from build123d import *

# Parameters (mm, degrees)
F1_DEPTH = 40
F3_DEPTH = 40
F5_DEPTH = 40
F7_DEPTH = 2


with BuildPart() as f1:
    # F0 (on Front) → F1 (new body)
    with BuildSketch(Plane.XZ):
        Polygon((-30, -33.600594), (-15, -7.619832), (-45, -7.619832), align=None)
        Polygon((-18.464102, -9.619832), (-30, -29.600594), (-41.535898, -9.619832), align=None, mode=Mode.SUBTRACT)
        Polygon((0, -33.600594), (-15, -7.619832), (-30, -33.600594), align=None)
        Polygon((-3.464102, -31.600594), (-26.535898, -31.600594), (-15, -11.619832), align=None, mode=Mode.SUBTRACT)
        Polygon((0, -33.600594), (15, -7.619832), (-15, -7.619832), align=None)
        Polygon((-11.535898, -9.619832), (11.535898, -9.619832), (0, -29.600594), align=None, mode=Mode.SUBTRACT)
        Polygon((-15, -7.619832), (15, -7.619832), (0, 18.360931), align=None)
        Polygon((-11.535898, -5.619832), (0, 14.360931), (11.535898, -5.619832), align=None, mode=Mode.SUBTRACT)
    extrude(amount=F1_DEPTH)

    # F2 (on face) → F3 (join)
    with BuildSketch(Plane.XZ.offset(40)):
        Polygon((-30, -33.600594), (-45, -7.619832), (-75, -7.619832), (-105, -7.619832), (-90, -33.600594), align=None)
        Polygon((-33.464102, -31.600594), (-88.845299, -31.600594), (-101.535898, -9.619832), (-75, -9.619832), (-46.154701, -9.619832), align=None, mode=Mode.SUBTRACT)
    extrude(amount=-F3_DEPTH)

    # F4 (on face) → F5 (join)
    with BuildSketch(Plane.XZ.offset(40)):
        Polygon((-75, -7.619832), (-90, 18.360931), (-105, -7.619832), align=None)
        Polygon((-101.535898, -5.619832), (-90, 14.360931), (-78.464102, -5.619832), (-90, -5.619832), align=None, mode=Mode.SUBTRACT)
    extrude(amount=-F5_DEPTH)

    # F6 (on face) → F7 (join)
    with BuildSketch(Plane(origin=(0, 0, 0), x_dir=(-1, 0, 0), z_dir=(0, 1, 0))):
        Polygon((0, 18.360931), (-15, -7.619832), (0, -33.600594), (90, -33.600594), (105, -7.619832), (90, 18.360931), (75, -7.619832), (15, -7.619832), align=None)
    extrude(amount=F7_DEPTH)


solid = f1.part
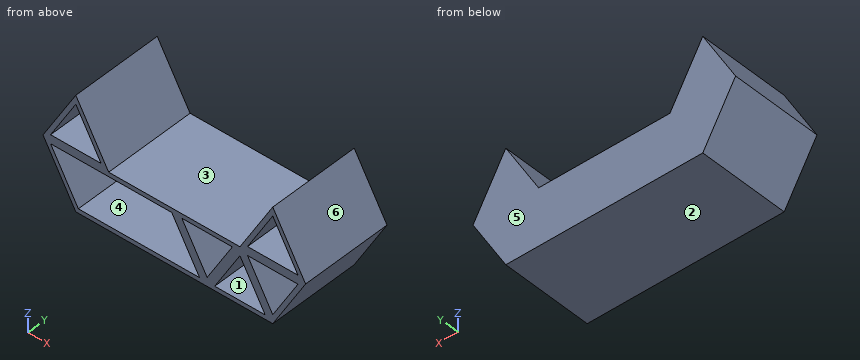
For this review, take the finished solid that the model builds, in its own axes (mm). Face numbers are marked on the shaded views. A direction names the side the tool comes from. Round coordinates to 2 decimals unless told otherwise and drop trailing zeros. Order: outer loops, then holes, each group sorted by start corner. A loop starts at its lowest first (then second) coordinate and runs counter-clockwise, first axis right, second up. Notation, with made-up numbers: M -11.5,19 L -5.5,19 A24 cw -5.5,42 Z; hole C 6,60.5 d5. An arc over 180 degrees is marked long. Write each question's results on one line, items separated by ' | '. Start each with the question number.
1. Add section D-D (z = 11.5). State the section outline as (x, y) points, then the cut area to 3 significant figures.
2. Add section C-C (x = -68). State the section outline as (y, z) points.
3. Clearance check with flat-ended pins moving along their axes: pin 1 Ø8 at (y, z) = (-29.5, 5) entering from -X; pin 2 Ø7 at (x, y) = (-86, -11) entering from +Z; pin 3 Ø12 at (x, y) = (-79, -27) entering from +Z. State where each tip first meets the part, or that it passes through.
4. Tool access review of the marked faces 1, 2 and 3: name each direction out of +Z, -Z, +X, -X, +Y, -Y from which nothing blocks a thin tool from reaching the whole face with its end or side.
5. Add section B-B (z = -3.5). State the section outline as (x, y) points.
6. To check wall thickness, follow L1, parallel to Z at x = -45, y = -29.5; L2, parallel to X at y = -15, z = -30; L3, parallel to Z at x = -58, y = -13. State the ranges of each line that lie inside material, in increasing order. Write a range as [from, to].
7. Add section A-A (y = -8.5). State the section outline as (x, z) points.
8. Draft analysis for pull direction X (two halves, no side actions). For the marked faces 4, 5 and 6, state which applies: pulls with the +X half, pulls with the -X half, needs draft (parallel to the pull), parting line crosses it, or undercut.
Output values:
1) outline: M -93.96,-40 L -91.65,-40 L -91.65,0 L -88.35,0 L -88.35,-40 L -86.04,-40 L -86.04,2 L -93.96,2 Z; M -3.96,-40 L -1.65,-40 L -1.65,0 L 1.65,0 L 1.65,-40 L 3.96,-40 L 3.96,2 L -3.96,2 Z | area: 401 mm^2
2) outline: M -40,-33.6 L 2,-33.6 L 2,-7.62 L -40,-7.62 L -40,-9.62 L 0,-9.62 L 0,-31.6 L -40,-31.6 Z
3) pin 1: x = -100.02 | pin 2: z = 17.49 | pin 3: z = 9.7
4) face 1: -Y | face 2: -Z, +X, -X, +Y, -Y | face 3: +Z, +Y, -Y
5) outline: M -102.62,-40 L -100.31,-40 L -100.31,0 L -79.69,0 L -79.69,-40 L -77.38,-40 L -77.38,2 L -102.62,2 Z; M -12.62,-40 L -10.31,-40 L -10.31,0 L 10.31,0 L 10.31,-40 L 12.62,-40 L 12.62,2 L -12.62,2 Z
6) L1: [-33.6, -31.6], [-11.62, -7.62] | L2: [-92.08, -89.77], [-34.39, -25.61], [-4.39, 2.08] | L3: [-33.6, -31.6], [-9.62, -7.62]
7) outline: M -105,-7.62 L -90,-33.6 L 0,-33.6 L 15,-7.62 L 0,18.36 L -15,-7.62 L -75,-7.62 L -90,18.36 Z; hole M -101.54,-9.62 L -88.85,-31.6 L -33.46,-31.6 L -46.15,-9.62 Z; hole M -101.54,-5.62 L -78.46,-5.62 L -90,14.36 Z; hole M -41.54,-9.62 L -30,-29.6 L -18.46,-9.62 Z; hole M -26.54,-31.6 L -3.46,-31.6 L -15,-11.62 Z; hole M -11.54,-9.62 L 0,-29.6 L 11.54,-9.62 Z; hole M -11.54,-5.62 L 11.54,-5.62 L 0,14.36 Z
8) face 4: undercut | face 5: needs draft | face 6: pulls with the +X half
